Source: CAD feature listing. Evaluate the final solid. Frame: model axes, mm. Face numbers are marked on the shaded views. Coordinates: 2 decimals unless noted, no trailing zeros. Order: outer loops, then holes, each group sorted by start corner. A loop starts at its lowest first (then second) coordinate and runs counter-clockwise, first axis right, second up.
Item 1: Section B-B on z = 12.5. Return the cut outline in (x, y), then the cut area to 3 significant figures.
Item 2: Mould query, pull axis Z, two halves, no side actions, for the marked faces 1, 2 and 3. Classes: released by +Z, released by -Z, zero draft, split by the parting line, or undercut.
Item 3: Ray query, line 1 (Z direction, x = -136, y = -8.25); line 2 (Z direction, x = 173, y = -21.5); line 3 (X direction, y = -28, z = -92). Return the intervals inside material, ascending.
Item 4: Contact query for flat-ended pins moving along their axis: P1, Ø4, axis at x = -45, z = 117, coming from the +Y side; P2, Ø0.6, axis at x = -132.5, z = -144.5, coming from the +Y side. Output: stop coordinate, or through.
Item 5: Section A-A on x = 114.5. Return the cut outline in (y, z).
from build123d import *

# Parameters (mm, degrees)
F0_W      = 412
F0_H      = 305
F1_DEPTH  = 30
F2_W      = 230
F2_H      = 275
F3_DEPTH  = 30
F4_R      = 3
F5_R      = 30
F6_W      = 26
F6_H      = 167
F7_DEPTH  = 3.5
F8_R      = 3
F10_W     = 32
F10_H     = 92
F11_DEPTH = 26
F12_R     = 3
F13_W     = 4
F13_H     = 47
F14_DEPTH = 20
F15_R     = 3
F16_W     = 30
F16_H     = 76.5
F17_DEPTH = 3
F18_R     = 2.99999
F19_R     = 3.5
F20_DEPTH = 30
F21_W     = 99
F21_H     = 62
F22_DEPTH = 18
F23_R     = 3
F25_DEPTH = 6
F26_W     = 13
F26_H     = 20
F26_H_2   = 6
F27_DEPTH = 30
F28_R     = 1
F29_DEPTH = 30
F31_DEPTH = 20


# Not quite as in the source:
# - a fillet or chamfer is up to 0.001 mm smaller than in the source, because OpenCascade refuses the exact size
# - a feature names something its author has since deleted; it is built from what else it names


with BuildPart() as f1:
    # F0 (on Front) → F1 (new body)
    with BuildSketch(Plane.XZ):
        Rectangle(F0_W, F0_H)
    extrude(amount=F1_DEPTH)

    # F2 (on face) → F3 (cut, through all)
    with BuildSketch(Plane.XZ.offset(30)):
        with Locations((67, 0)):
            Rectangle(F2_W, F2_H)
    extrude(amount=-F3_DEPTH, mode=Mode.SUBTRACT)

    # F4
    f4_edges = [f1.edges().sort_by_distance(p)[0] for p in [
        (-48, -15, 137.5),
        (182, -15, 137.5),
        (182, -15, -137.5),
        (-48, -15, -137.5),
    ]]
    fillet(f4_edges, radius=F4_R)

    # F5
    f5_edges = [f1.edges().sort_by_distance(p)[0] for p in [
        (-206, -15, -152.5),
        (-206, -15, 152.5),
        (206, -15, 152.5),
        (206, -15, -152.5),
    ]]
    fillet(f5_edges, radius=F5_R)

    # F6 (on face) → F7 (cut)
    with BuildSketch(Plane.YZ.offset(-48)):
        with Locations((-13, 35.5)):
            Rectangle(F6_W, F6_H)
    extrude(amount=-F7_DEPTH, mode=Mode.SUBTRACT)

    # F8
    f8_edges = [f1.edges().sort_by_distance(p)[0] for p in [
        (-51.5, -13, -48),
        (-51.5, -13, 119),
    ]]
    fillet(f8_edges, radius=F8_R)

    # F10 (on face) → F11 (cut)
    with BuildSketch(Plane(origin=(0, 0, 0), x_dir=(-1, 0, 0), z_dir=(0, 1, 0))):
        with Locations((67.5, 31.5)):
            Rectangle(F10_W, F10_H)
    extrude(amount=-F11_DEPTH, mode=Mode.SUBTRACT)

    # F12
    f12_edges = [f1.edges().sort_by_distance(p)[0] for p in [
        (-83.5, -13, -14.5),
        (-83.5, -13, 77.5),
    ]]
    fillet(f12_edges, radius=F12_R)

    # F13 (on face) → F14 (cut)
    with BuildSketch(Plane.YZ.offset(-48)):
        with Locations((-28, 43)):
            Rectangle(F13_W, F13_H)
    extrude(amount=-F14_DEPTH, mode=Mode.SUBTRACT)

    # F15
    f15_edges = [f1.edges().sort_by_distance(p)[0] for p in [
        (-68, -28, 19.5),
        (-68, -28, 66.5),
    ]]
    fillet(f15_edges, radius=F15_R)

    # F16 (on face) → F17 (cut)
    with BuildSketch(Plane(origin=(182, 0, 0), x_dir=(0, -1, 0), z_dir=(-1, 0, 0))):
        with Locations((15, -66.25)):
            Rectangle(F16_W, F16_H)
        with Locations((15, 66.25)):
            Rectangle(F16_W, F16_H)
    extrude(amount=-F17_DEPTH, mode=Mode.SUBTRACT)

    # F18 (radius 3 in the source; OpenCascade refuses exactly that, so slightly less here)
    f18_edges = [f1.edges().sort_by_distance(p)[0] for p in [
        (185, -15, -104.5),
        (185, -15, 28),
        (185, -15, 104.5),
        (185, -15, -28),
    ]]
    fillet(f18_edges, radius=F18_R)

    # F19 (on face) → F20 (cut)
    with BuildSketch(Plane.XZ.offset(30)):
        with Locations((-136, -23.25)):
            Circle(F19_R)
    extrude(amount=-F20_DEPTH, mode=Mode.SUBTRACT)

    # F21 (on face) → F22 (cut)
    with BuildSketch(Plane(origin=(0, 0, 0), x_dir=(-1, 0, 0), z_dir=(0, 1, 0))):
        with Locations((126.5, -97.75)):
            Rectangle(F21_W, F21_H)
    extrude(amount=-F22_DEPTH, mode=Mode.SUBTRACT)

    # F23
    f23_edges = [f1.edges().sort_by_distance(p)[0] for p in [
        (-176, -9, -128.75),
        (-77, -9, -128.75),
        (-77, -9, -66.75),
        (-176, -9, -66.75),
    ]]
    fillet(f23_edges, radius=F23_R)

    # F24 (on face) → F25 (cut)
    with BuildSketch(Plane(origin=(0, 0, 0), x_dir=(-1, 0, 0), z_dir=(0, 1, 0))):
        with BuildLine():
            ThreePointArc((139.5, -23.25), (136, -26.75), (132.5, -23.25))
            Line((132.5, -23.25), (132.5, -66.75))
            Line((132.5, -66.75), (139.5, -66.75))
            Line((139.5, -66.75), (139.5, -23.25))
        make_face()
    extrude(amount=-F25_DEPTH, mode=Mode.SUBTRACT)

    # F26 (on face) → F27 (cut)
    with BuildSketch(Plane(origin=(-206, 0, 0), x_dir=(0, -1, 0), z_dir=(-1, 0, 0))):
        with Locations((6.5, -92.5)):
            Rectangle(F26_W, F26_H)
        with Locations((6.5, -113.5)):
            Rectangle(F26_W, F26_H_2)
    extrude(amount=-F27_DEPTH, mode=Mode.SUBTRACT)

    # F28 (on face) → F29 (cut)
    with BuildSketch(Plane.XZ.offset(30)):
        with Locations((-158.5, 75.35)):
            Circle(F28_R)
        with Locations((-158.5, -41.25)):
            Circle(F28_R)
        with Locations((-113.5, -41.25)):
            Circle(F28_R)
        with Locations((-113.5, 75.35)):
            Circle(F28_R)
    extrude(amount=-F29_DEPTH, mode=Mode.SUBTRACT)

    # F30 (on face) → F31 (cut)
    with BuildSketch(Plane(origin=(0, 0, 0), x_dir=(-1, 0, 0), z_dir=(0, 1, 0))):
        with BuildLine():
            Line((-194, 120), (-194, 122))
            ThreePointArc((-194, 122), (-195, 121), (-194, 120))
        make_face()
        with BuildLine():
            ThreePointArc((-193, 121), (-193.2928932188, 121.7071067812), (-194, 122))
            Line((-194, 122), (-194, 120))
            ThreePointArc((-194, 120), (-193.2928932188, 120.2928932188), (-193, 121))
        make_face()
        with BuildLine():
            ThreePointArc((-68, 145), (-67, 144), (-66, 145))
            Line((-66, 145), (-68, 145))
        make_face()
        with BuildLine():
            Line((-68, 145), (-66, 145))
            ThreePointArc((-66, 145), (-67, 146), (-68, 145))
        make_face()
        with BuildLine():
            Line((131.5, 145), (133.5, 145))
            ThreePointArc((133.5, 145), (132.5, 146), (131.5, 145))
        make_face()
        with BuildLine():
            ThreePointArc((131.5, 145), (132.5, 144), (133.5, 145))
            Line((133.5, 145), (131.5, 145))
        make_face()
        with BuildLine():
            ThreePointArc((192, 0), (191.7071067812, 0.7071067812), (191, 1))
            Line((191, 1), (191, -1))
            ThreePointArc((191, -1), (191.7071067812, -0.7071067812), (192, 0))
        make_face()
        with BuildLine():
            Line((191, -1), (191, 1))
            ThreePointArc((191, 1), (190, 0), (191, -1))
        make_face()
        with BuildLine():
            Line((131.5, -145), (133.5, -145))
            ThreePointArc((133.5, -145), (132.5, -144), (131.5, -145))
        make_face()
        with BuildLine():
            ThreePointArc((131.5, -145), (132.5, -146), (133.5, -145))
            Line((133.5, -145), (131.5, -145))
        make_face()
        with BuildLine():
            Line((-68, -145), (-66, -145))
            ThreePointArc((-66, -145), (-67, -144), (-68, -145))
        make_face()
        with BuildLine():
            ThreePointArc((-68, -145), (-67, -146), (-66, -145))
            Line((-66, -145), (-68, -145))
        make_face()
        with BuildLine():
            ThreePointArc((-193, -121), (-193.2928932188, -120.2928932188), (-194, -120))
            Line((-194, -120), (-194, -122))
            ThreePointArc((-194, -122), (-193.2928932188, -121.7071067812), (-193, -121))
        make_face()
        with BuildLine():
            Line((-194, -122), (-194, -120))
            ThreePointArc((-194, -120), (-195, -121), (-194, -122))
        make_face()
        with BuildLine():
            Line((-194, -1), (-194, 1))
            ThreePointArc((-194, 1), (-195, 0), (-194, -1))
        make_face()
        with BuildLine():
            ThreePointArc((-193, 0), (-193.2928932188, 0.7071067812), (-194, 1))
            Line((-194, 1), (-194, -1))
            ThreePointArc((-194, -1), (-193.2928932188, -0.7071067812), (-193, 0))
        make_face()
    extrude(amount=-F31_DEPTH, mode=Mode.SUBTRACT)


solid = f1.part
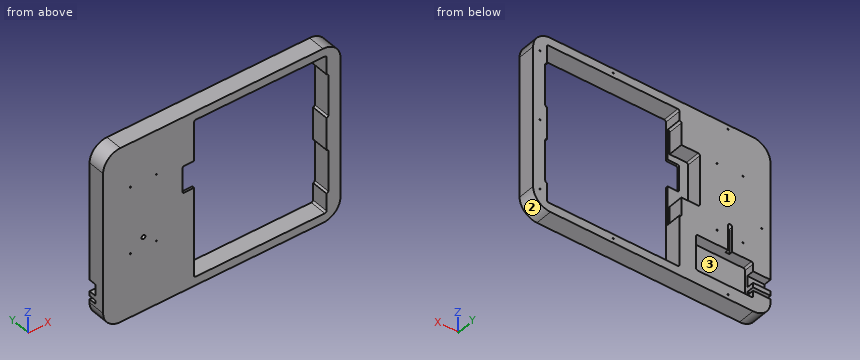
Answer list:
1. outline: (-206, -30) - (-48, -30) - (-48, -26) - (-83.5, -26) - (-83.5, 0) - (-206, 0) - close; (182, -30) - (206, -30) - (206, 0) - (182, 0) - close
1. area: 4,540 mm2
2. face 1: zero draft
2. face 2: released by -Z
2. face 3: undercut
3. line 1: z = -152.5 to -128.75, -66.75 to -26.75, -19.75 to 152.5
3. line 2: z = -152.5 to -137.5, 137.5 to 152.5
3. line 3: x = -206 to -48, 185 to 206
4. P1: passes through
4. P2: stops at y = -20
5. outline: (-30, -152.5) - (0, -152.5) - (0, -137.5) - (-30, -137.5) - close; (-30, 137.5) - (0, 137.5) - (0, 152.5) - (-30, 152.5) - close
